Read the model definition and answer for the solid it produces. Units are mm, in the model's axes. Face numbers are marked on the shaded views. Coordinates: 2 decimals unless noted, no trailing zeros. Order: outer loops, then holes, each group sorted by start corner. A loop starts at its lowest first (then second) coordinate and runs counter-clockwise, first axis right, second up. Notation, with made-up numbers: (42, 73.5) -> (67, 73.5) arc R36 cw to (67, 112.5) -> close; hole circle Ø3 at (32, -31). An arc over 180 degrees is marked (long way). Answer in a Markdown table with one row per item.
from build123d import *

# Parameters (mm, degrees)
F0_W     = 178.507768
F0_H     = 91.6887
F1_DEPTH = 6.35
F2_R     = 5.08
F3_T     = -2.54


with BuildPart() as f1:
    # F0 (on Top) → F1 (new body)
    with BuildSketch(Plane.XY):
        with Locations((-30.921195, -4.082151)):
            Rectangle(F0_W, F0_H)
    extrude(amount=F1_DEPTH)

    # F2
    f2_edges = [f1.edges().sort_by_distance(p)[0] for p in [
        (-30.921195, -49.926501, 6.35),
        (-30.921195, 41.762199, 6.35),
        (-120.175079, -4.082151, 6.35),
        (58.332689, -4.082151, 6.35),
    ]]
    fillet(f2_edges, radius=F2_R)

    # F3
    f3_openings = [f1.faces().sort_by_distance(p)[0] for p in [
        (-30.921195, -4.082151, 0),
    ]]
    offset(amount=F3_T, openings=f3_openings)


solid = f1.part
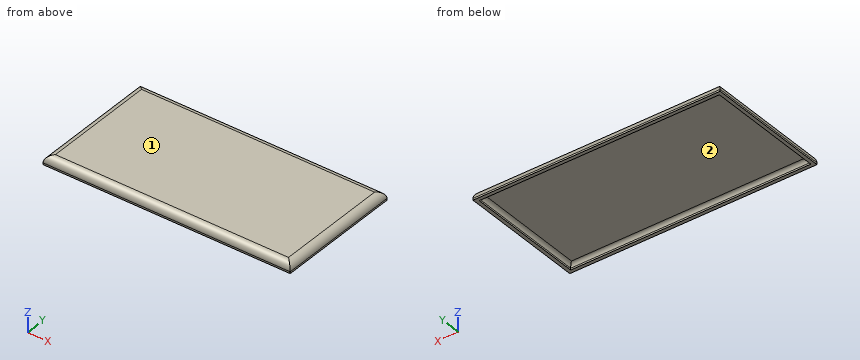
Q1. The part is cut by section C-C (y = -30). Write down the section's boundary in (x, z), then the cut area to 3 significant figures.
Outcome:
| item | result |
|---|---|
| outline | (-120.18, 0) -> (-117.64, 0) -> (-117.64, 1.27) arc R2.54 cw to (-115.1, 3.81) -> (53.25, 3.81) arc R2.54 cw to (55.79, 1.27) -> (55.79, 0) -> (58.33, 0) -> (58.33, 1.27) arc R5.08 ccw to (53.25, 6.35) -> (-115.1, 6.35) arc R5.08 ccw to (-120.18, 1.27) -> close |
| area | 464 mm² |
Q2. Consider line 1 (X direction, y = 28, z = 0.75); line 2 (Y direction, x = -97.5, z = 1); line 3 (X direction, y = 19, z = 3). Determine where each line is inside the solid, lowest interval first.
Outcome:
| item | result |
|---|---|
| line 1 | -120.18 to -117.64, 55.79 to 58.33 |
| line 2 | -49.93 to -47.39, 39.22 to 41.76 |
| line 3 | -119.87 to -116.95, 55.11 to 58.03 |
Q3. The part is cut by section B-B (z = 2.25). Write down the section's boundary in (x, y).
Outcome:
| item | result |
|---|---|
| outline | (-120.08, -49.83) -> (58.24, -49.83) -> (58.24, 41.67) -> (-120.08, 41.67) -> close; hole (-117.44, -47.19) -> (55.6, -47.19) -> (55.6, 39.03) -> (-117.44, 39.03) -> close |
Q4. Given pin 1 (4 mm diameter, centred on x = -1, y = -2, fed in from -Z); pin 2 (1.5 mm diameter, centred on y = 13.5, z = 2.5, fed in from +X); pin 3 (3 mm diameter, centred on x = -71.5, z = 5.5, fed in from +Y), each flat-ended and moving along its own axis, determine where each tip first touches the part or whether it passes through.
Outcome:
| item | result |
|---|---|
| pin 1 | z = 3.81 |
| pin 2 | x = 58.31 |
| pin 3 | y = 40.97 |
Q5. The part is cut by section A-A (x = -17.5). Write down the section's boundary in (y, z), then the cut area to 3 significant figures.
Outcome:
| item | result |
|---|---|
| outline | (-49.93, 0) -> (-47.39, 0) -> (-47.39, 1.27) arc R2.54 cw to (-44.85, 3.81) -> (36.68, 3.81) arc R2.54 cw to (39.22, 1.27) -> (39.22, 0) -> (41.76, 0) -> (41.76, 1.27) arc R5.08 ccw to (36.68, 6.35) -> (-44.85, 6.35) arc R5.08 ccw to (-49.93, 1.27) -> close |
| area | 244 mm² |
Q6. For a pull along Y with two mould halves and no side action, classify the marked faces 1 and 2 as pulls with the +Y half, pulls with the -Y half, needs draft (parallel to the pull), parting line crosses it, or undercut.
Outcome:
| item | result |
|---|---|
| face 1 | needs draft |
| face 2 | undercut |
